from build123d import *

# Parameters (mm, degrees)
SKETCH1_R           = 5.75
BOSS_EXTRUDE1_DEPTH = 14.5
BOSS_EXTRUDE1_TAPER = 1
FILLET1_R           = 1
FILLET2_R           = 0.5
CUT_EXTRUDE1_DEPTH  = 7


with BuildPart() as part:
    # Sketch1 → Boss-Extrude1 (new body)
    with BuildSketch(Plane(origin=(0, 0, 0), x_dir=(1, 0, 0), z_dir=(0, 1, 0))):
        Circle(SKETCH1_R)
    extrude(amount=BOSS_EXTRUDE1_DEPTH, taper=BOSS_EXTRUDE1_TAPER)

    # Fillet1
    fillet1_edges = [part.edges().sort_by_distance(p)[0] for p in [
        (-5.496901559, 14.5, 0),
    ]]
    fillet(fillet1_edges, radius=FILLET1_R)

    # Fillet2
    fillet2_edges = [part.edges().sort_by_distance(p)[0] for p in [
        (-5.75, 0, 0),
    ]]
    fillet(fillet2_edges, radius=FILLET2_R)

    # Sketch2 → Cut-Extrude1 (cut)
    with BuildSketch(Plane.XZ):
        with BuildLine():
            Line((2.598076211, -1.5), (-2.598076211, -1.5))
            ThreePointArc((-2.598076211, -1.5), (0, 3), (2.598076211, -1.5))
        make_face()
    extrude(amount=-CUT_EXTRUDE1_DEPTH, mode=Mode.SUBTRACT)


solid = part.part
Design review of the part built by this model. Coordinates are the model's own, in mm. A direction names the side the tool comes from. Coordinates: 2 decimals unless noted, no trailing zeros. Order: outer loops, then holes, each group sorted by start corner. A loop starts at its lowest first (then second) coordinate and runs counter-clockwise, first axis right, second up. Notation, with made-up numbers: (40, -38.75) -> (66, -38.75) arc R35 ccw to (66, -5.75) -> close; hole circle Ø7 at (-19, 23). An arc over 180 degrees is marked (long way). Use one line per item in the form item = value. Start each with the question number.
(1) Add section A-A on y = 1.5. State the section outline as (x, z) points.
(2) For faces 4 (the flat face through (0, 3, -1.5)), 5 (the flat face through (0, 0, -2)), list the 3-axis set-ups (+Z, -Z, +X, -X, +Y, -Y) from which the entire face can be reached by the end or side of a thin tool; tool diameter is ignored.
(3) Add section B-B on y = 12.5. State the section outline as (x, z) points.
(4) Add section C-C on y = 6.5. State the section outline as (x, z) points, plus the area to 3 significant figures.
(5) Insertion check: pin 1 (1.3 mm diameter, centred on x = -0.5, z = 1, fed in from -Y); pin 2 (3 mm diameter, centred on x = -1.5, y = 4, fed in from +Z); pin 3 (5 mm diameter, centred on x = 2.5, y = 9, fed in from -Z). Each pin has a flat end and moves straight along its axis. Give the tip position at first contact, or say it passes through.
(6) For probe 1 along Y at (x, z) = (-0.5, -0.25); probe 2 along Z at (x, y) = (-1, 6.75); probe 3 along X at (y, z) = (4.75, 2.75), list the stretches that pass through material, from the lowest coordinate up.
(7) The part is to be moulded in two halves that separate along X. For faces 1 (the cylindrical face through (0, 3, 3)), 2 (the flat face through (0, 14.5, 0)), 3 (the conical face through (-1.22, 7.104, 5.492)), say which applies: +X half, -X half, draft (parallel to the pull), parting line (faces both ways), or undercut.
Answer block:
q1.outline = circle Ø11.45 at (0, 0); hole (-2.6, -1.5) -> (2.6, -1.5) arc R3 ccw (long way) to start
q2.face_4 = -Y
q2.face_5 = +Z, -Z, +X, -X, -Y
q3.outline = circle Ø11.06 at (0, 0)
q4.outline = circle Ø11.27 at (0, 0); hole (-2.6, -1.5) -> (2.6, -1.5) arc R3 ccw (long way) to start
q4.area = 77.1 mm²
q5.pin_1 = 7
q5.pin_2 = 5.69
q5.pin_3 = -5.61
q6.probe_1 = 7 to 14.5
q6.probe_2 = -5.54 to -1.5, 2.83 to 5.54
q6.probe_3 = -4.96 to -1.2, 1.2 to 4.96
q7.face_1 = undercut
q7.face_2 = draft
q7.face_3 = parting line
